from build123d import *

# Parameters (mm, degrees)
SKETCH1_W                                           = 246
SKETCH1_H                                           = 36.2
EXTRUDE1_DEPTH                                      = 78
HOLE3_D                                             = 40
LPATTERN1_COUNT                                     = 2
LPATTERN1_PITCH                                     = 180
M6_TAPPED_HOLE1_D                                   = 5
HOLE4_D                                             = 8
M8_TAPPED_HOLE1_D                                   = 6.8
LPATTERN2_COUNT                                     = 2
LPATTERN2_PITCH                                     = 100
LPATTERN2_COUNT_DIR2                                = 2
LPATTERN2_PITCH_DIR2                                = 156
M6_TAPPED_HOLE2_D                                   = 5
M6_TAPPED_HOLE3_D                                   = 5
LPATTERN3_COUNT                                     = 2
LPATTERN3_PITCH                                     = 135
LPATTERN3_COUNT_DIR2                                = 2
LPATTERN3_PITCH_DIR2                                = 120
HOLE6_D                                             = 10
HOLE6_DEPTH                                         = 25
SKETCH30_R                                          = 2.5
CUT_EXTRUDE1_DEPTH                                  = 37.2
SKETCH31_R                                          = 5
CUT_EXTRUDE2_DEPTH                                  = 24.2
CBORE_FOR_M3_HEX_SOCKET_HEAD_CAP_SCREW1_D           = 3.4
CBORE_FOR_M3_HEX_SOCKET_HEAD_CAP_SCREW1_CBORE_D     = 6.5
CBORE_FOR_M3_HEX_SOCKET_HEAD_CAP_SCREW1_CBORE_DEPTH = 6.4
CBORE_FOR_M4_HEX_SOCKET_HEAD_CAP_SCREW1_D           = 4.5
CBORE_FOR_M4_HEX_SOCKET_HEAD_CAP_SCREW1_CBORE_D     = 8
CBORE_FOR_M4_HEX_SOCKET_HEAD_CAP_SCREW1_CBORE_DEPTH = 4.4
CUT_EXTRUDE3_DEPTH                                  = 8


with BuildPart() as part:
    # Sketch1 → Extrude1 (new body, symmetric)
    with BuildSketch(Plane.XY):
        with Locations((0, 18.1)):
            Rectangle(SKETCH1_W, SKETCH1_H)
    extrude(amount=EXTRUDE1_DEPTH, both=True)

    # Hole3 (through all)
    with Locations(Plane.XZ):
        with Locations((90, 0)):
            hole3 = Hole(HOLE3_D / 2)

    # LPattern1: Hole3 ×2
    with Locations(*[(-i * LPATTERN1_PITCH, 0, 0) for i in range(1, LPATTERN1_COUNT)]):
        add(hole3, mode=Mode.SUBTRACT)

    # M6 Tapped Hole1 (through all)
    with Locations(Plane(origin=(0, 36.2, 0), x_dir=(-1, 0, 0), z_dir=(0, 1, 0))):
        with Locations((-40, 35), (40, 35), (40, -35), (-40, -35)):
            Hole(M6_TAPPED_HOLE1_D / 2)

    # Hole4 (through all)
    with Locations(Plane(origin=(0, 36.2, 0), x_dir=(-1, 0, 0), z_dir=(0, 1, 0))):
        with Locations((-40, -53), (-40, 53), (40, 53), (40, -53)):
            Hole(HOLE4_D / 2)

    # M8 Tapped Hole1 (through all)
    with Locations(Plane(origin=(0, 36.2, 0), x_dir=(-1, 0, 0), z_dir=(0, 1, 0))):
        with Locations((78, 50)):
            m8_tapped_hole1 = Hole(M8_TAPPED_HOLE1_D / 2)

    # LPattern2: M8 Tapped Hole1 2 × 2
    with Locations(*[(j * LPATTERN2_PITCH_DIR2, 0, -i * LPATTERN2_PITCH) for i in range(LPATTERN2_COUNT) for j in range(LPATTERN2_COUNT_DIR2) if (i, j) != (0, 0)]):
        add(m8_tapped_hole1, mode=Mode.SUBTRACT)

    # M6 Tapped Hole2 (through all)
    with Locations(Plane(origin=(0, 36.2, 0), x_dir=(-1, 0, 0), z_dir=(0, 1, 0))):
        with Locations((90, 30), (90, -30), (-90, -30), (-90, 30)):
            Hole(M6_TAPPED_HOLE2_D / 2)

    # M6 Tapped Hole3 (through all)
    with Locations(Plane(origin=(0, 36.2, 0), x_dir=(-1, 0, 0), z_dir=(0, 1, 0))):
        with Locations((67.5, -60)):
            m6_tapped_hole3 = Hole(M6_TAPPED_HOLE3_D / 2)

    # LPattern3: M6 Tapped Hole3 2 × 2
    with Locations(*[(i * LPATTERN3_PITCH, 0, j * LPATTERN3_PITCH_DIR2) for i in range(LPATTERN3_COUNT) for j in range(LPATTERN3_COUNT_DIR2) if (i, j) != (0, 0)]):
        add(m6_tapped_hole3, mode=Mode.SUBTRACT)

    # Hole6
    with Locations(Plane(origin=(0, 36.2, 0), x_dir=(-1, 0, 0), z_dir=(0, 1, 0))):
        with Locations((-12.15, 35), (12.15, 35), (-12.15, 5), (12.15, 5), (14.65, 14), (-14.65, 14), (-14.65, 44), (14.65, 44)):
            Hole(HOLE6_D / 2, depth=HOLE6_DEPTH)

    # Sketch30 → Cut-Extrude1 (cut, through all)
    with BuildSketch(Plane(origin=(0, 36.2, 0), x_dir=(1, 0, 0), z_dir=(0, 1, 0))):
        with Locations((-1.269390874, -5)):
            Circle(SKETCH30_R)
        with BuildLine():
            Line((3.104640419, 59), (-4.895359581, 59))
            ThreePointArc((-4.895359581, 59), (-8.895359581, 63), (-4.895359581, 67))
            Line((-4.895359581, 67), (3.104640419, 67))
            ThreePointArc((3.104640419, 67), (7.104640419, 63), (3.104640419, 59))
        make_face()
        with BuildLine():
            Line((16.96, 11.01), (0.696577832, 11.01))
            ThreePointArc((0.696577832, 11.01), (-0.010528949, 10.717106781), (-0.303422168, 10.01))
            Line((-0.303422168, 10.01), (-0.303422168, 3.99))
            ThreePointArc((-0.303422168, 3.99), (-0.010528949, 3.282893219), (0.696577832, 2.99))
            Line((0.696577832, 2.99), (16.96, 2.99))
            ThreePointArc((16.96, 2.99), (17.667106781, 3.282893219), (17.96, 3.99))
            Line((17.96, 3.99), (17.96, 10.01))
            ThreePointArc((17.96, 10.01), (17.667106781, 10.717106781), (16.96, 11.01))
        make_face()
        with BuildLine():
            Line((-3.235359581, 11.01), (-16.735359581, 11.01))
            ThreePointArc((-16.735359581, 11.01), (-17.442466362, 10.717106781), (-17.735359581, 10.01))
            Line((-17.735359581, 10.01), (-17.735359581, 3.99))
            ThreePointArc((-17.735359581, 3.99), (-17.442466362, 3.282893219), (-16.735359581, 2.99))
            Line((-16.735359581, 2.99), (-3.235359581, 2.99))
            ThreePointArc((-3.235359581, 2.99), (-2.5282528, 3.282893219), (-2.235359581, 3.99))
            Line((-2.235359581, 3.99), (-2.235359581, 10.01))
            ThreePointArc((-2.235359581, 10.01), (-2.5282528, 10.717106781), (-3.235359581, 11.01))
        make_face()
    extrude(amount=-CUT_EXTRUDE1_DEPTH, mode=Mode.SUBTRACT)

    # Sketch31 → Cut-Extrude2 (cut)
    with BuildSketch(Plane.XZ):
        with Locations((-1.269390874, 5)):
            Circle(SKETCH31_R)
    extrude(amount=-CUT_EXTRUDE2_DEPTH, mode=Mode.SUBTRACT)

    # CBORE for M3 Hex Socket Head Cap Screw1 (through all)
    with Locations(Plane.XZ):
        with Locations((-12.195359581, -21), (12.4, -21), (0.904640419, -36.5), (6.904640419, -41.5)):
            CounterBoreHole(CBORE_FOR_M3_HEX_SOCKET_HEAD_CAP_SCREW1_D / 2, CBORE_FOR_M3_HEX_SOCKET_HEAD_CAP_SCREW1_CBORE_D / 2, CBORE_FOR_M3_HEX_SOCKET_HEAD_CAP_SCREW1_CBORE_DEPTH)

    # CBORE for M4 Hex Socket Head Cap Screw1 (through all)
    with Locations(Plane.XZ):
        with Locations((-25, -7), (25, -7), (-13.395359581, -63), (11.604640419, -63)):
            CounterBoreHole(CBORE_FOR_M4_HEX_SOCKET_HEAD_CAP_SCREW1_D / 2, CBORE_FOR_M4_HEX_SOCKET_HEAD_CAP_SCREW1_CBORE_D / 2, CBORE_FOR_M4_HEX_SOCKET_HEAD_CAP_SCREW1_CBORE_DEPTH)

    # Sketch36 → Cut-Extrude3 (cut)
    with BuildSketch(Plane(origin=(0, 36.2, 0), x_dir=(1, 0, 0), z_dir=(0, 1, 0))):
        with BuildLine():
            Line((17.25, 46.6), (-17.25, 46.6))
            ThreePointArc((-17.25, 46.6), (-19.371320344, 45.721320344), (-20.25, 43.6))
            Line((-20.25, 43.6), (-20.25, 18.4))
            ThreePointArc((-20.25, 18.4), (-19.371320344, 16.278679656), (-17.25, 15.4))
            Line((-17.25, 15.4), (17.25, 15.4))
            ThreePointArc((17.25, 15.4), (19.371320344, 16.278679656), (20.25, 18.4))
            Line((20.25, 18.4), (20.25, 43.6))
            ThreePointArc((20.25, 43.6), (19.371320344, 45.721320344), (17.25, 46.6))
        make_face()
    extrude(amount=-CUT_EXTRUDE3_DEPTH, mode=Mode.SUBTRACT)


solid = part.part
For this review, take the finished solid that the model builds, in its own axes (mm). A direction names the side the tool comes from. Round coordinates to 2 decimals unless told otherwise and drop trailing zeros. Loops run counter-clockwise (first coordinate to the right, second up) from the corner with the lowest first, then second, coordinate; pieces in that order, holes last. Notation, with made-up numbers: (39, 89.25) - (58, 89.25) arc R26 cw to (58, 122.25) - close; hole circle Ø10 at (36, -23). An arc over 180 degrees is marked (long way). Use one line per item in the form item = value.
1) Clearance check with flat-ended pins moving along their axes: P1, Ø5.5, axis at x = 12.4, z = -21, coming from the +Y side; P2, Ø5, axis at x = 25, z = -7, coming from the -Y side; P3, Ø5, axis at x = 0.9, z = -36.5, coming from the -Y side. State where each tip first meets the part, or that it passes through.
Solutions:
P1 = 28.2
P2 = 4.4
P3 = 6.4
2) Wall thickness on probe 1 along Z at (x, y) = (-25, 2.5); probe 2 along X at (y, z) = (22.5, -49.5); probe 3 along X at (y, z) = (17, 39): over which ranges is each line inside the solid? List them lowest first.
Solutions:
probe_1 = -78 to -11, -3 to 78
probe_2 = -123 to -81.36, -74.64 to -41.94, -38.06 to 38.06, 41.94 to 74.64, 81.36 to 123
probe_3 = -123 to -15.15, -9.15 to 9.15, 15.15 to 123
3) We need section A-A on z = -30. Write out the cut boundary in (x, y).
Solutions:
outline = (-123, 0) - (-92.5, 0) - (-92.5, 36.2) - (-123, 36.2) - close; (-87.5, 0) - (87.5, 0) - (87.5, 36.2) - (20.25, 36.2) - (20.25, 28.2) - (-20.25, 28.2) - (-20.25, 36.2) - (-87.5, 36.2) - close; (92.5, 0) - (123, 0) - (123, 36.2) - (92.5, 36.2) - close
4) We need section C-C on y = 32. State how many separate pieces and enclosed holes the cut face has, then the cut area to 3 significant figures.
Solutions:
separate_pieces = 1
enclosed_holes = 35
area = 32,900 mm2
5) We need section B-B on z = 5. Write out the cut boundary in (x, y), then the cut area to 3 significant figures.
Solutions:
outline = (-123, 0) - (-109.36, 0) - (-109.36, 36.2) - (-123, 36.2) - close; (-70.64, 0) - (-6.27, 0) - (-6.27, 24.2) - (-3.77, 24.2) - (-3.77, 36.2) - (-7.15, 36.2) - (-7.15, 11.2) - (-17.15, 11.2) - (-17.15, 36.2) - (-70.64, 36.2) - close; (1.23, 24.2) - (3.73, 24.2) - (3.73, 0) - (70.64, 0) - (70.64, 36.2) - (17.15, 36.2) - (17.15, 11.2) - (7.15, 11.2) - (7.15, 36.2) - (1.23, 36.2) - close; (109.36, 0) - (123, 0) - (123, 36.2) - (109.36, 36.2) - close
area = 5,300 mm2
6) Mouldability with a two-part tool opening along X and no side actions: class faces 4 (the face through (-2, 0, 18)), 5 (the face through (-70.02, 18.35, 0.88)) as pulls with the +X half, pulls with the -X half, needs draft (parallel to the pull), parting line crosses it, or undercut.
Solutions:
face_4 = needs draft
face_5 = undercut
7) Tool access review of faces 1 (the face through (-15.8, 23.525, 48.866)), 2 (the face through (-0.303, 18, -7)), 3 (the face through (21.8, 2.2, -9.4)): name each direction out of +Z, -Z, +X, -X, +Y, -Y from which nothing blocks a thin tool from reaching the whole face with its end or side.
Solutions:
face_1 = +Y
face_2 = +Y, -Y
face_3 = -Y
